from build123d import *

# Parameters (mm, degrees)
F2_R = 0.2


with BuildPart() as f1:
    # F0 (on Front) → F1 (revolve)
    with BuildSketch(Plane.XZ):
        with BuildLine():
            Line((2.5, 5.2), (0, 5.2))
            Line((0, 5.2), (0, 0))
            Line((0, 0), (2.5, 0))
            Line((2.5, 0), (2.5, 1))
            ThreePointArc((2.5, 1), (2.3, 1.2), (2.5, 1.4))
            Line((2.5, 1.4), (2.5, 5.2))
        make_face()
    revolve(axis=Axis((0, 0, 6.706364), (0, 0, -1)))

    # F2
    f2_edges = [f1.edges().sort_by_distance(p)[0] for p in [
        (-2.5, 0, 1.4),
        (-2.5, 0, 1),
        (-2.5, 0, 5.2),
    ]]
    fillet(f2_edges, radius=F2_R)


solid = f1.part
Work out the finished part from the listing and answer in its coordinate system (mm). Give positions to 0.01 mm unless a question says otherwise; leave off trailing zeros. Loops run counter-clockwise (first coordinate to the right, second up) from the corner with the lowest first, then second, coordinate; pieces in that order, holes last. Notation, with made-up numbers: (-25.75, 15) -> (-13.75, 15) arc R27 ccw to (-13.75, 38) -> close; hole circle Ø5 at (35, -20.75). An arc over 180 degrees is marked (long way). Use a Markdown table: item, result. Add a question column.
1) For a pull along Y with two mould halves and no side action, classify faces 1 (the flat face through (0, 0, 0)), 2 (the cylindrical face through (-0.54, 2.44, 0.43)) as +Y half, -Y half, draft (parallel to the pull), parting line (faces both ways), or undercut.
2) The part is cut by section A-A, the plane z = 2.95. Determine the outline of the cut face in (x, y), plus the area to 3 significant figures.
3) Consider line 1 along X through (y, z) = (0.1, 3.05); line 2 along Y through (x, z) = (-0.8, 4.75); line 3 along Y through (x, z) = (1.9, 1.6). Determine where each line is inside the solid, lowest interval first.
4) This flat-tipped pin is pushed along its axis until it touches: P1, Ø2, axis at x = -1.5, z = 3.5, coming from the +Y side. Where does it stop, or does it pass through?
Reported:
| question | item | result |
|---|---|---|
| 1 | face 1 | draft |
| 1 | face 2 | parting line |
| 2 | outline | circle Ø5 at (0, 0) |
| 2 | area | 19.6 mm^2 |
| 3 | line 1 | x = -2.5 to 2.5 |
| 3 | line 2 | y = -2.37 to 2.37 |
| 3 | line 3 | y = -1.62 to 1.62 |
| 4 | P1 | stops at y = 2.45 |
